Input: part model. Units: mm. Frame: model coordinates. A direction names the side the tool comes from. Round coordinates to 2 decimals unless told otherwise and drop trailing zeros. Write each loop counter-clockwise with the first axis right and the second up, starting at its lowest first coordinate (ties: lowest second). Pieces come first, ordered by that corner, then holes. Notation, with made-up numbers: (46, 44) -> (79, 44) arc R17 cw to (79, 61) -> close; hole circle Ø8 at (88.5, 16). An arc over 180 degrees is marked (long way). Use CSV: the item, a comma, the result in double quotes.
```python
from build123d import *

# Parameters (mm, degrees)
VERRUNDUNG1_R = 1
FASE1_SIZE    = 0.5
VERRUNDUNG2_R = 1


with BuildPart() as part:
    # Skizze1 → Rotation1 (revolve)
    with BuildSketch(Plane.XY, mode=Mode.PRIVATE) as rotation1_sk:
        Polygon((0, -40.15), (0, -45.424522078), (45, -46.21), (45, -36.5), (41, -36.5), (41, -24.25), (9.17986928, -24.25), align=None)
    revolve(rotation1_sk.sketch.rotate(Axis((0, 0, 0), (1, 0, 0)), 270), axis=Axis((0, 0, 0), (1, 0, 0)))  # turned: the seam where the file's is

    # Verrundung1
    verrundung1_edges = [part.edges().sort_by_distance(p)[0] for p in [
        (45, 0, -46.21),
        (0, 0, -45.424522078),
    ]]
    fillet(verrundung1_edges, radius=VERRUNDUNG1_R)

    # Fase1
    fase1_edges = [part.edges().sort_by_distance(p)[0] for p in [
        (41, 0, -24.25),
        (45, 0, -36.5),
    ]]
    chamfer(fase1_edges, length=FASE1_SIZE)

    # Verrundung2
    verrundung2_edges = [part.edges().sort_by_distance(p)[0] for p in [
        (41, 0, -36.5),
    ]]
    fillet(verrundung2_edges, radius=VERRUNDUNG2_R)


solid = part.part
```
Item 1: Line query: line 1 (X direction, y = -25, z = 37); line 2 (Y direction, x = 31, z = 11); line 3 (Z direction, x = 39.5, y = -6). Output: solid intervals per line, ascending.
Worked answers:
line 1,"x = 0.02 to 45"
line 2,"y = -44.63 to -21.61, 21.61 to 44.63"
line 3,"z = -45.72 to -23.5, 23.5 to 45.72"
Item 2: Pull-direction query (Y, two-part tool) for faces 3 (the face through (45, 33.3, -16.9)), 4 (the face through (43.232, 35.632, -7.912)), 5 (the face through (22.784, 44.733, -9.933)); classes: +Y half, -Y half, draft (parallel to the pull), parting line (faces both ways), or undercut.
Worked answers:
face 3,"draft"
face 4,"undercut"
face 5,"parting line"
Item 3: Section query B-B on x = 29. Return the cut outline in (y, z).
Worked answers:
outline,"circle Ø91.86 at (0, 0); hole circle Ø48.5 at (0, 0)"
Item 4: Section query A-A on x = 22. Return the cut outline in (y, z).
Worked answers:
outline,"circle Ø91.62 at (0, 0); hole circle Ø48.5 at (0, 0)"
Item 5: Set-up query: faces 1 (the face through (41, 7, -24)), 2 (the face through (24.621, 21.514, 11.19)). Return all of +Z, -Z, +X, -X, +Y, -Y with unobstructed straight access to the full face (end or side cutting, diameter ignored); none if empty.
Worked answers:
face 1,"+X"
face 2,"+X, -X"
Item 6: First-contact query: pin 1 Ø1.5 at (y, z) = (29.5, 7) entering from +X; pin 2 Ø2 at (y, z) = (20, -17.5) entering from -X; pin 3 Ø5 at (y, z) = (-29.5, 14.5) entering from -X; pin 4 Ø4 at (y, z) = (-4.5, 21) entering from -X. Flat tips, straight axial feed; report the tip coordinate or a pass-through.
Worked answers:
pin 1,"stops at x = 41"
pin 2,"stops at x = 7.26"
pin 3,"stops at x = 2.76"
pin 4,"passes through"
